Here's the drawing with two shaded views (mm, measured from the low corner). I have some questions. Coordinates: 2 decimals unless noted, no trailing zeros. Order: outer loops, then holes, each group sorted by start corner. A loop starts at its lowest first (then second) coordinate and runs counter-clockwise, first axis right, second up. Notation, with made-up numbers: (89, 1) -> (111, 1) arc R18 cw to (111, 11) -> close; hole circle Ø3 at (87.5, 74.5). An arc over 180 degrees is marked (long way). Answer in a Markdown table with one row per item. Add a question column.
1. Imagine slicing it at D-D on x = 78. Write out the boundary of the cut face in (y, z) (1 decimal).
2. If I drill on line 1 along Y through (x, z) = (6, 49); line 2 along X through (y, z) = (7, 6.5); line 3 along Z through (x, y) = (115, 5.5) (1 decimal), over which ranges is the centre line in solid material (lowest first)? Write a range as [from, to].
3. Imagine slicing it at B-B on x = 99. Write out the boundary of the cut face in (y, z), plus the area to 3 significant figures.
4. Will these pins go through, and if not, where does the flat tip stop? pin 1 (12 mm diameter, centred on y = 20, z = 27, fed in from -X); pin 2 (3 mm diameter, centred on x = 24.5, y = 5, fed in from -Z); pin 3 (5 mm diameter, centred on y = 3, z = 12.5, fed in from -X); pin 4 (4 mm diameter, centred on x = 63.5, z = 47, fed in from -Y).
5. We'd pull the mould along X, two halves only. Please class the marked faces 1 and 2: pulls with the +X half, pulls with the -X half, needs draft (parallel to the pull), parting line crosses it, or undercut.
6. Imagine slicing it at A-A on y = 10.25. State how many separate pieces and enclosed holes the cut face has, plus the area to 3 significant figures.
7. Imagine slicing it at C-C on z = 79. Write out the boundary of the cut face in (x, y) (1 decimal).
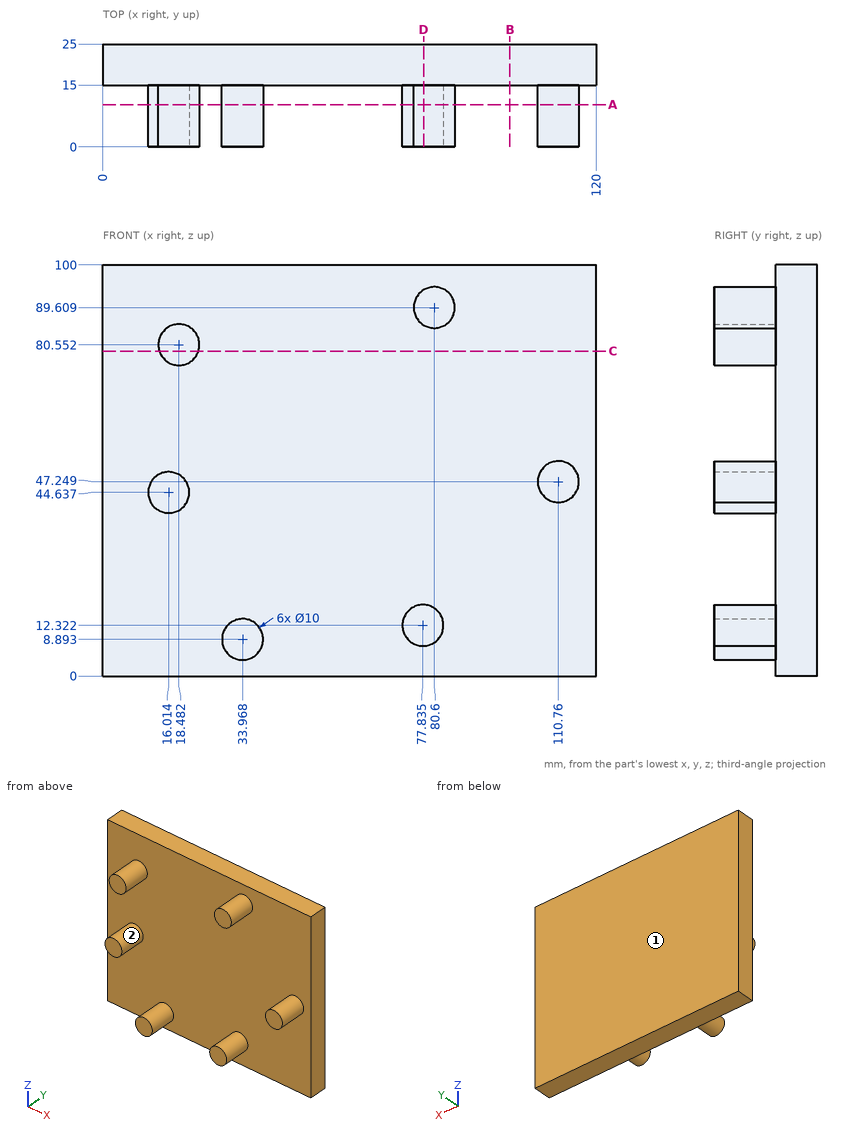
Answers follow:
| question | item | result |
|---|---|---|
| 1 | outline | (0, 7.3) -> (15, 7.3) -> (15, 0) -> (25, 0) -> (25, 100) -> (15, 100) -> (15, 93.9) -> (0, 93.9) -> (0, 85.3) -> (15, 85.3) -> (15, 17.3) -> (0, 17.3) -> close |
| 2 | line 1 | y = [15, 25] |
| 2 | line 2 | x = [29.58, 38.36] |
| 2 | line 3 | z = [44.6, 49.9] |
| 3 | outline | (15, 0) -> (25, 0) -> (25, 100) -> (15, 100) -> close |
| 3 | area | 1,000 mm² |
| 4 | pin 1 | stops at x = 0 |
| 4 | pin 2 | stops at z = 78.41 |
| 4 | pin 3 | stops at x = 29.09 |
| 4 | pin 4 | stops at y = 15 |
| 5 | face 1 | needs draft |
| 5 | face 2 | undercut |
| 6 | separate pieces | 6 |
| 6 | enclosed holes | 0 |
| 6 | area | 471 mm² |
| 7 | outline | (0, 15) -> (13.7, 15) -> (13.7, 0) -> (23.2, 0) -> (23.2, 15) -> (120, 15) -> (120, 25) -> (0, 25) -> close |
